Build history of the part. All positions in model axes, mm. Coordinates: 2 decimals unless noted, no trailing zeros. Loops run counter-clockwise (first coordinate to the right, second up) from the corner with the lowest first, then second, coordinate; pieces in that order, holes last.
Item 1: Cut at C-C (x = 2). List the corners of the cut face in (y, z).
Item 2: Cut at B-B (z = -5). List the corners of the cut face in (x, y), and give its area (3 significant figures).
Item 3: Cut at D-D (x = -2). List the corners of the cut face in (y, z).
Item 4: Mould opens along Z. For faces 1 (the face through (1, 0, -45.5)), 2 (the face through (-1.95, -0.21, -6.2)), 3 (the face through (1.74, 7.83, -22.43)) say: released by +Z, released by -Z, zero draft, split by the parting line, or undercut.
Item 5: Cut at A-A (y = -9). List the corners of the cut face in (x, z), and give its area (3 significant figures).
Item 6: Drill centre lines: line 1 along Y through (x, z) = (2, -22.5); line 2 along X through (y, z) = (-3.5, -5); line 3 along X through (y, z) = (-9, -25.5). Where is each one in solid material? Low to high.
from build123d import *

# Parameters (mm, degrees)
ESQUISSE1_W             = 12
ESQUISSE1_H             = 45.5
ESQUISSE1_R             = 1.2
BOSS_EXTRU_1_DEPTH      = 15
ESQUISSE2_R             = 1.2
ENL_V_MAT_EXTRU_1_DEPTH = 49.28301979
CONG_1_R                = 3


with BuildPart() as part:
    # Esquisse1 → Boss.-Extru.1 (new, symmetric)
    with BuildSketch(Plane(origin=(0, 0, 0), x_dir=(1, 0, 0), z_dir=(0, 1, 0))):
        with Locations((0, 22.75)):
            Rectangle(ESQUISSE1_W, ESQUISSE1_H)
        with Locations(Location((-2, 5, 0), (0, 0, 270))):
            Circle(ESQUISSE1_R, mode=Mode.SUBTRACT)
    extrude(amount=BOSS_EXTRU_1_DEPTH, both=True)

    # Esquisse2 → Enlèv. mat.-Extru.1 (cut, through all)
    with BuildSketch(Plane.XY):
        with Locations((2, 9)):
            Circle(ESQUISSE2_R)
        with Locations(Location((2, -9, 0), (0, 0, 180))):
            Circle(ESQUISSE2_R)
    extrude(amount=-ENL_V_MAT_EXTRU_1_DEPTH, mode=Mode.SUBTRACT)

    # Congé1
    cong_1_edges = [part.edges().sort_by_distance(p)[0] for p in [
        (-6, 0, -45.5),
        (-6, 0, 0),
    ]]
    fillet(cong_1_edges, radius=CONG_1_R)


solid = part.part
Filled sheet:
1. outline: (-15, -45.5) - (-10.2, -45.5) - (-10.2, 0) - (-15, 0) - close; (-7.8, -45.5) - (7.8, -45.5) - (7.8, 0) - (-7.8, 0) - close; (10.2, -45.5) - (15, -45.5) - (15, 0) - (10.2, 0) - close
2. outline: (-6, -15) - (-3.2, -15) - (-3.2, 15) - (-6, 15) - close; (-0.8, -15) - (6, -15) - (6, 15) - (-0.8, 15) - close; hole circle Ø2.4 at (2, -9); hole circle Ø2.4 at (2, 9)
2. area: 279 mm2
3. outline: (-15, -45.5) - (15, -45.5) - (15, -6.2) - (-15, -6.2) - close; (-15, -3.8) - (15, -3.8) - (15, 0) - (-15, 0) - close
4. face 1: released by -Z
4. face 2: undercut
4. face 3: zero draft
5. outline: (-6, -42.5) arc R3 ccw to (-3, -45.5) - (0.8, -45.5) - (0.8, 0) - (-3, 0) arc R3 ccw to (-6, -3) - close; (3.2, -45.5) - (6, -45.5) - (6, 0) - (3.2, 0) - close; hole circle Ø2.4 at (-2, -5)
5. area: 428 mm2
6. line 1: y = -15 to -10.2, -7.8 to 7.8, 10.2 to 15
6. line 2: x = -6 to -3.2, -0.8 to 6
6. line 3: x = -6 to 0.8, 3.2 to 6
